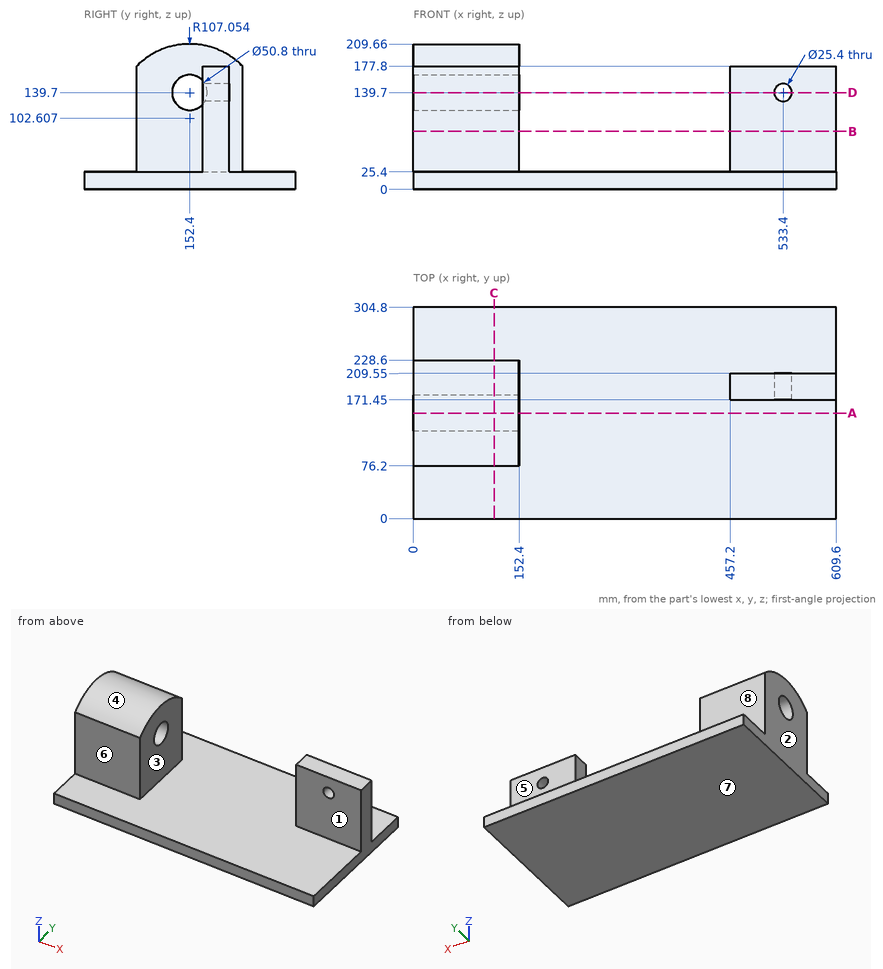
Design review of the part shown in the three views and the two pictorial views. Dimensions are in mm from the part's minimum x, y and z. A direction names the side the tool comes from. Give positions to 0.01 mm unless a question says otherwise; leave off trailing zeros. Loops run counter-clockwise (first coordinate to the right, second up) from the corner with the lowest first, then second, coordinate; pieces in that order, holes last. Notation, with made-up numbers: (83, 68) -> (103, 68) arc R5 ccw to (103, 75) -> close; hole circle Ø8 at (-10.75, 19). An arc over 180 degrees is marked (long way). Answer as a JSON object with one key per item and string values. Group by question number.
Q1. Take a section at B-B (z = 83.5). Write out the cut boundary in (x, y), plus the area to 3 significant figures.
Q2. Tool access review of the marked faces 4, 5, 6, 7 and 8: name each direction out of +Z, -Z, +X, -X, +Y, -Y from which nothing blocks a thin tool from reaching the whole face with its end or side.
Q3. Take a section at A-A (y = 152.4). Write out the cut boundary in (x, z).
Q4. Insertion check: pin 1 (5 mm diameter, centred on x = 247.5, y = 131.5, fed in from -Z); pin 2 (4 mm diameter, centred on x = 284, y = 87.5, fed in from +Z). Each pin has a flat end and moves straight along its axis. Give the tip position at first contact, or say it passes through.
Q5. Draft analysis for pull direction X (two halves, no side actions). For the marked faces 1, 2 and 3, state which applies: pulls with the +X half, pulls with the -X half, needs draft (parallel to the pull), parting line crosses it, or undercut.
Q6. Take a section at C-C (x = 116.5). Write out the cut boundary in (y, z), plus the area to 3 significant figures.
Q7. Wall thickness on line 1 along Z through (x, y) = (533, 198); line 2 along X through (y, z) = (202, 176); line 3 along Z through (x, y) = (52, 152): over which ranges is each line inside the solid? List them lowest first.
Q8. Take a section at D-D (z = 139.7). Write out the cut boundary in (x, y), plus the area to 3 significant figures.
Answer below:
{
 "1": {"outline": "(0, 76.2) -> (152.4, 76.2) -> (152.4, 228.6) -> (0, 228.6) -> close; (457.2, 171.45) -> (609.6, 171.45) -> (609.6, 209.55) -> (457.2, 209.55) -> close", "area": "29,000 mm2"},
 "2": {"face 4": "+Z, +X, -X", "face 5": "+Z, +X, +Y", "face 6": "+Z, +X, -X, -Y", "face 7": "-Z, +X, -X, +Y, -Y", "face 8": "+Z, +X, -X, +Y"},
 "3": {"outline": "(0, 0) -> (609.6, 0) -> (609.6, 25.4) -> (152.4, 25.4) -> (152.4, 114.3) -> (0, 114.3) -> close; (0, 165.1) -> (152.4, 165.1) -> (152.4, 209.66) -> (0, 209.66) -> close"},
 "4": {"pin 1": "stops at z = 0", "pin 2": "stops at z = 25.4"},
 "5": {"face 1": "needs draft", "face 2": "pulls with the -X half", "face 3": "undercut"},
 "6": {"outline": "(0, 0) -> (304.8, 0) -> (304.8, 25.4) -> (228.6, 25.4) -> (228.6, 177.8) arc R107.05 ccw to (76.2, 177.8) -> (76.2, 25.4) -> (0, 25.4) -> close; hole circle Ø50.8 at (152.4, 139.7)", "area": "32,300 mm2"},
 "7": {"line 1": "z = 0 to 127.01, 152.39 to 177.8", "line 2": "x = 0 to 152.4, 457.2 to 609.6", "line 3": "z = 0 to 114.3, 165.1 to 209.66"},
 "8": {"outline": "(0, 76.2) -> (152.4, 76.2) -> (152.4, 127) -> (0, 127) -> close; (0, 177.8) -> (152.4, 177.8) -> (152.4, 228.6) -> (0, 228.6) -> close; (457.2, 171.45) -> (520.7, 171.45) -> (520.7, 209.55) -> (457.2, 209.55) -> close; (546.1, 171.45) -> (609.6, 171.45) -> (609.6, 209.55) -> (546.1, 209.55) -> close", "area": "20,300 mm2"}
}
